Design review of the part shown in the three views and the two pictorial views. Dimensions are in mm from the part's minimum x, y and z. Coordinates: 2 decimals unless noted, no trailing zeros. Loops run counter-clockwise (first coordinate to the right, second up) from the corner with the lowest first, then second, coordinate; pieces in that order, holes last. Notation, with made-up numbers: (-38.75, -30) -> (18.25, -30) arc R27 cw to (18.25, 6) -> close; hole circle Ø11 at (45.5, 80.25). An arc over 180 degrees is marked (long way). One line per item, written item: value. Start each with the question number.
1. Add section B-B on y = 19.25. Write out the cut boundary in (x, z) (3 decimals).
2. Add section C-C on y = 3.75. Write out the cut boundary in (x, z) (3 decimals).
3. Add section A-A on z = 0.7. Write out the cut boundary in (x, y) (3 decimals), plus the area to 3 significant figures.
4. Insertion check: pin 1 (1.6 mm diameter, centred on x = 11.825, y = 17.36, fed in from -Z); pin 2 (1.5 mm diameter, centred on y = 5.5, z = 1.5, fed in from -X). Each pin has a flat end and moves straight along its axis. Give the tip position at first contact, or say it passes through.
5. For probe 1 along X at (y, z) = (16.75, 1.4) (3 decimals); probe 2 along X at (y, z) = (7, 0.4) (3 decimals); probe 3 along X at (y, z) = (18.25, 1.65) (3 decimals), list the stretches that pass through material, from the lowest coordinate up.
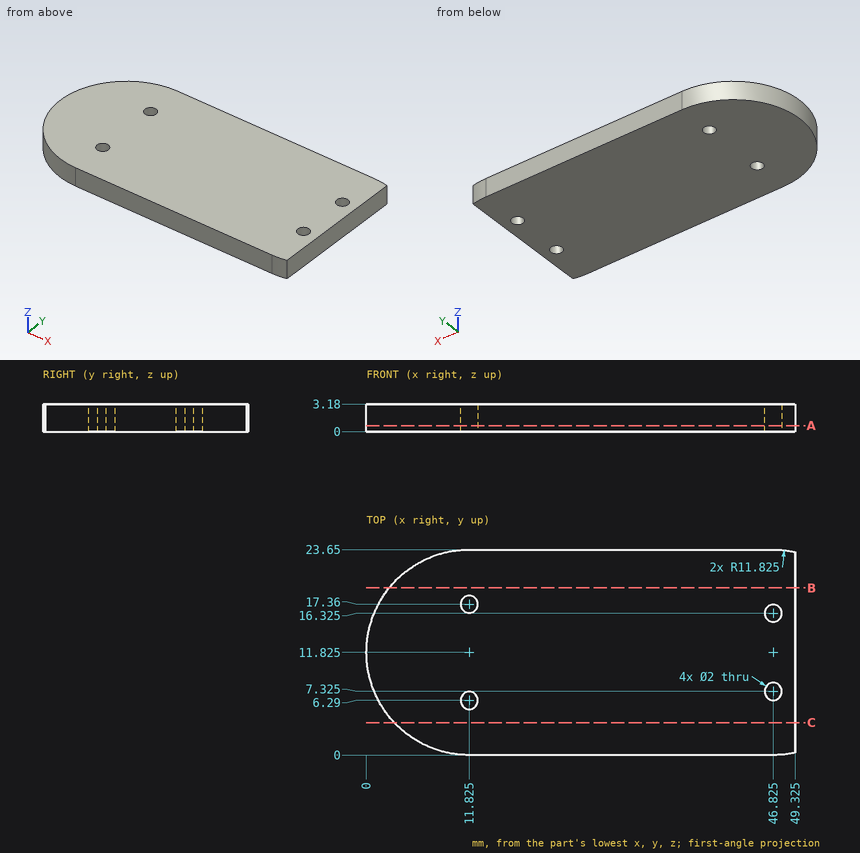
Worked answers:
1. outline: (2.622, 0) -> (49.325, 0) -> (49.325, 3.18) -> (2.622, 3.18) -> close
2. outline: (3.186, 0) -> (49.325, 0) -> (49.325, 3.18) -> (3.186, 3.18) -> close
3. outline: (11.825, 0) -> (46.825, 0) arc R11.825 ccw to (49.325, 0.267) -> (49.325, 23.383) arc R11.825 ccw to (46.825, 23.65) -> (11.825, 23.65) arc R11.825 ccw to start; hole circle Ø2 at (11.825, 6.29); hole circle Ø2 at (11.825, 17.36); hole circle Ø2 at (46.825, 7.325); hole circle Ø2 at (46.825, 16.325)
3. area: 1,090 mm²
4. pin 1: passes through
4. pin 2: stops at x = 1.4
5. probe 1: x = 1.074 to 11.033, 12.617 to 45.92, 47.73 to 49.325
5. probe 2: x = 1.029 to 11.121, 12.529 to 45.879, 47.771 to 49.325
5. probe 3: x = 1.898 to 11.369, 12.281 to 49.325
